Geometry check sheet. Reference: drawing and pictorial views, mm from the part's lowest x, y, z. Give positions to 0.01 mm unless a question says otherwise; leave off trailing zeros. Loops run counter-clockwise (first coordinate to the right, second up) from the corner with the lowest first, then second, coordinate; pieces in that order, holes last. Notation, with made-up numbers: M 86,10 L 98,10 A4 ccw 98,15 Z; hole C 79.5,22.5 d7. An arc over 180 degrees is marked long. Use CSV: the item, a comma, the result in double quotes.
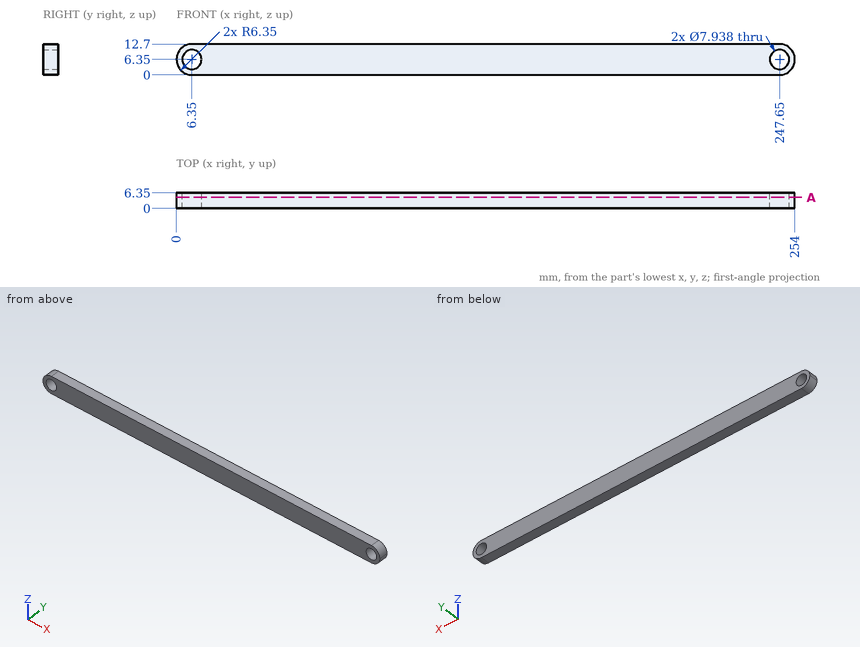
(1) Section check A-A on y = 4.5. Record the cut outline in (x, z).
Calculated:
outline,"M 6.35,0 L 247.65,0 A6.35 ccw 247.65,12.7 L 6.35,12.7 A6.35 ccw Z; hole C 6.35,6.35 d7.94; hole C 247.65,6.35 d7.94"
(2) Scan lines: L1, parallel to X at y = 3.25, z = 9.75 (1 decimal); L2, parallel to X at y = 2.25, z = 4; L3, parallel to Z at x = 247.65, y = 2.75. Record each from-to range of solid material in increasing order. Write a range as from..to.
Calculated:
L1,"x = 1..4.3, 8.4..245.6, 249.7..253"
L2,"x = 0.45..3.15, 9.55..244.45, 250.85..253.55"
L3,"z = 0..2.38, 10.32..12.7"
(3) Depth check by flat-ended pin: pin 1 Ø2 at (y, z) = (1, 2) entering from +X (1 decimal); pin 2 Ø3 at (y, z) = (2.5, 11) entering from -X (1 decimal). Enter the tip coordinate at first touch or a pass-through.
Calculated:
pin 1,"stops at x = 253"
pin 2,"stops at x = 0.8"
